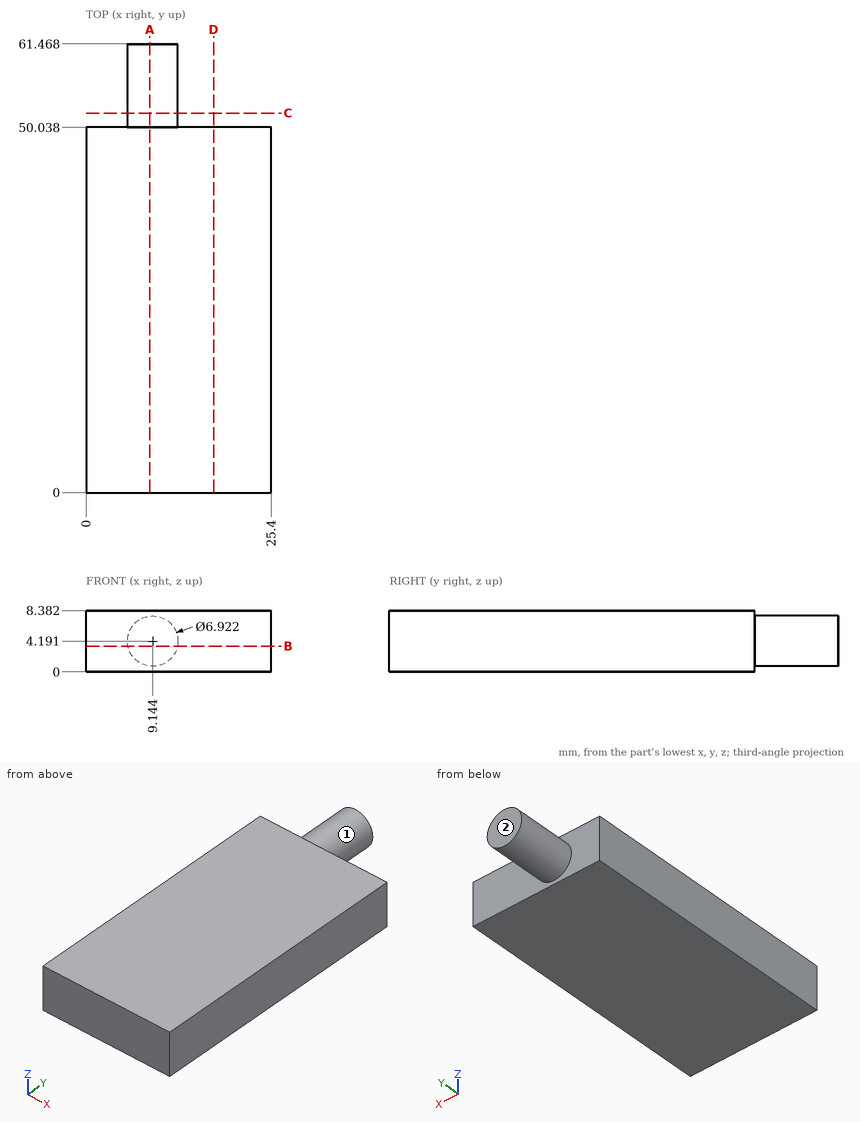
Drawing for the job (mm, zero at the part's lowest x, y, z). A direction names the side the tool comes from. Give positions to 0.01 mm unless a question says otherwise; leave off trailing zeros. Write each loop counter-clockwise with the first axis right and the second up, starting at its lowest first coordinate (ties: lowest second). Pieces come first, ordered by that corner, then holes. Notation, with made-up numbers: M 80.5,-5.75 L 116.5,-5.75 A8 cw 116.5,8.25 Z; hole C 21,13.5 d8. An arc over 180 degrees is marked long. Return JSON: item names as keys, results as strings. Group by question number.
(1) Band-saw the part on B-B (z = 3.5). Give the cut face in (x, y).
(2) 3-axis set-ups, long thin cutter, end or side, ignore diameter. For the marked faces 1 and 2: which of +Z, -Z, +X, -X, +Y, -Y reach the whole face in a straight line?
(3) Drill centre lines: L1, parallel to Y at x = 18.5, z = 2.75; L2, parallel to X at y = 54, z = 4; L3, parallel to X at y = 51, z = 1 (1 decimal). Where is each one in solid material? Low to high. Write a range as [from, to].
(4) Band-saw the part on D-D (x = 17.5). Give the cut face in (y, z).
(5) Band-saw the part on A-A (x = 8.75). Give the cut face in (y, z).
(6) Band-saw the part on C-C (y = 52). Give the cut face in (x, z) (1 decimal), and give its area (3 significant figures).
Entries:
{
 "1": {"outline": "M 0,0 L 25.4,0 L 25.4,50.04 L 12.54,50.04 L 12.54,61.47 L 5.75,61.47 L 5.75,50.04 L 0,50.04 Z"},
 "2": {"face 1": "+Y", "face 2": "+Z, -Z, +X, -X, +Y"},
 "3": {"L1": "y = [0, 50.04]", "L2": "x = [5.69, 12.6]", "L3": "x = [7.8, 10.5]"},
 "4": {"outline": "M 0,0 L 50.04,0 L 50.04,8.38 L 0,8.38 Z"},
 "5": {"outline": "M 0,0 L 50.04,0 L 50.04,0.75 L 61.47,0.75 L 61.47,7.63 L 50.04,7.63 L 50.04,8.38 L 0,8.38 Z"},
 "6": {"outline": "C 9.1,4.2 d6.9", "area": "37.6 mm^2"}
}
